Check sheet for the modelled part. Datum: model origin and axes. Units: mm. Face numbers are marked on the shaded views. A direction names the side the tool comes from. Round coordinates to 2 decimals unless told otherwise and drop trailing zeros. Order: outer loops, then holes, each group sorted by start corner. A loop starts at its lowest first (then second) coordinate and runs counter-clockwise, first axis right, second up.
```python
from build123d import *

# Parameters (mm, degrees)
ESBO_O1_R                = 1.6
RESSALTO_EXTRUS_O1_DEPTH = 6
RESSALTO_EXTRUS_O2_DEPTH = 6
FILETE1_R                = 10


with BuildPart() as part:
    # Esboço1 → Ressalto-extrusão1 (new body)
    with BuildSketch(Plane.XZ.offset(12)):
        with BuildLine():
            Line((-5.554408486, -1.950425304), (-0.098401843, -6.33585476))
            Line((-0.098401843, -6.33585476), (-0.098401843, -23.434191187))
            ThreePointArc((-0.098401843, -23.434191187), (0.884517689, -24.84224935), (2.545101876, -24.404963685))
            ThreePointArc((2.545101876, -24.404963685), (6.090429059, -19.835978921), (9.220727662, -14.973243345))
            ThreePointArc((9.220727662, -14.973243345), (9.728380083, -13.758965882), (9.901598157, -12.454291119))
            Line((9.901598157, -12.454291119), (9.901598157, -3.939806958))
            ThreePointArc((9.901598157, -3.939806958), (9.410602928, -1.779048764), (8.034047768, -0.042659356))
            Line((8.034047768, -0.042659356), (0.710490736, 5.843869901))
            ThreePointArc((0.710490736, 5.843869901), (-6.319106477, 5.07917191), (-5.554408486, -1.950425304))
        make_face()
        Circle(ESBO_O1_R, mode=Mode.SUBTRACT)
    extrude(amount=-RESSALTO_EXTRUS_O1_DEPTH)

    # Esboço2 → Ressalto-extrusão2 (add)
    with BuildSketch(Plane.XZ.offset(12)):
        with BuildLine():
            ThreePointArc((2.545101876, -24.404963685), (0.884517689, -24.84224935), (-0.098401843, -23.434191187))
            Line((-0.098401843, -23.434191187), (-0.098401843, -29.434191187))
            ThreePointArc((-0.098401843, -29.434191187), (0.598477482, -30.387143367), (1.71783387, -30.011910201))
            Line((1.71783387, -30.011910201), (9.901598157, -18.449402273))
            Line((9.901598157, -18.449402273), (9.901598157, -12.454291119))
            ThreePointArc((9.901598157, -12.454291119), (9.728380083, -13.758965882), (9.220727662, -14.973243345))
            ThreePointArc((9.220727662, -14.973243345), (6.090429059, -19.835978921), (2.545101876, -24.404963685))
        make_face()
    extrude(amount=-RESSALTO_EXTRUS_O2_DEPTH)

    # Filete1
    filete1_edges = [part.edges().sort_by_distance(p)[0] for p in [
        (9.901598157, -9, -18.449402273),
    ]]
    fillet(filete1_edges, radius=FILETE1_R)


solid = part.part
```
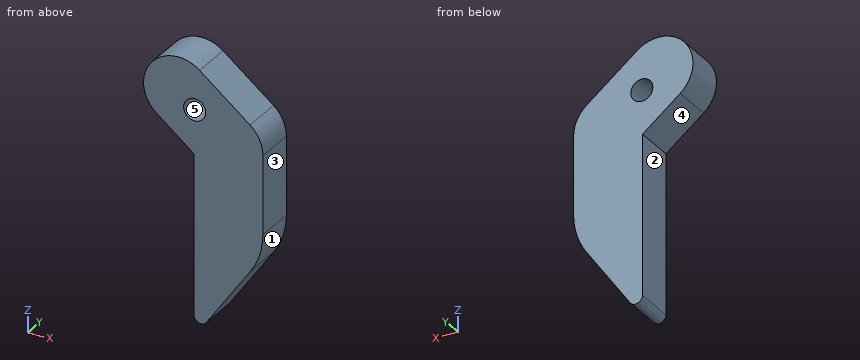
Item 1: Sectioned sample at B-B (z = -7). Record the cut outline in (x, y), and give its area (3 significant figures).
Answer:
outline: (-0.1, -12) - (9.9, -12) - (9.9, -6) - (-0.1, -6) - close
area: 60.0 mm2
Item 2: Go/stop test with flat-tipped pins: P1, Ø1, axis at x = -4, y = -7, coming from the +Z side; P2, Ø3, axis at x = 4.5, y = -11.5, coming from the +Z side; P3, Ø1.8, axis at y = -9.5, z = -15.5, coming from the -X side; P4, Ø2.5, axis at x = 0, z = 0, coming from the +Y side. Record where each tip stops, or that it passes through.
Answer:
P1: stops at z = 6.83
P2: stops at z = 4
P3: stops at x = -0.1
P4: passes through
Item 3: Access from +Z, -Z, +X, -X, +Y, -Y to the whole of each face (thin tool, end or side, straight path). Record for the marked faces 1 and 2.
Answer:
face 1: -Z, +X, +Y, -Y
face 2: -Z, -X, +Y, -Y
Item 4: Sectioned sample at C-C (x = 3.75). Record the cut outline in (y, z).
Answer:
outline: (-12, -27.14) - (-6, -27.14) - (-6, 3.4) - (-12, 3.4) - close
Item 5: Release check for a two-part mould opening along X. For the marked faces 3, 4 and 5 record: released by +X, released by -X, zero draft, split by the parting line, or undercut.
Answer:
face 3: released by +X
face 4: released by -X
face 5: undercut
Item 6: Scan lines: line 1 along X through (y, z) = (-11.45, -10.5); line 2 along Z through (x, y) = (0, -8.9); line 3 along X through (y, z) = (-10.9, -20). Record each from-to range of solid material in increasing order.
Answer:
line 1: x = -0.1 to 9.9
line 2: z = -29.87 to -1.6, 1.6 to 6.32
line 3: x = -0.1 to 8.71
Item 7: Sectioned sample at A-A (y = -6.65). Record the cut outline in (x, z), and give its area (3 significant figures).
Answer:
outline: (-5.55, -1.95) - (-0.1, -6.34) - (-0.1, -29.43) arc R1 ccw to (1.72, -30.01) - (8.06, -21.05) arc R10 ccw to (9.9, -15.27) - (9.9, -3.94) arc R5 ccw to (8.03, -0.04) - (0.71, 5.84) arc R5 ccw to start; hole circle Ø3.2 at (0, 0)
area: 337 mm2
